Work out the finished part from the listing and answer in its coordinate system (mm). Give positions to 0.01 mm unless a question says otherwise; leave off trailing zeros. Loops run counter-clockwise (first coordinate to the right, second up) from the corner with the lowest first, then second, coordinate; pieces in that order, holes last. Notation, with made-up numbers: M 64,14.5 L 94,14.5 A20 ccw 94,42.5 Z; hole C 71.25,62 d2. An arc over 180 degrees is marked long. Write item = value, one per line. Start each with the question number.
1. Section C-C on y = -67.5 is taken. Determine the outline of the cut face in (x, z), plus the area to 3 significant figures.
2. Consider L1, parallel to X at y = -32.5, z = -9; L2, parallel to Z at x = -26, y = -16; L3, parallel to X at y = -8.5, z = -20. Determine where each line is inside the solid, lowest interval first. Write a range as [from, to].
3. Section D-D on x = 19 is taken. Determine the outline of the cut face in (y, z).
4. Flat-ended cylindrical pins translate along their axes: pin 1 Ø12 at (x, z) = (10, 13.5) entering from +Y; pin 2 Ø1.5 at (x, y) = (-49, -57.5) entering from +Z; pin 3 Ø5 at (x, y) = (41, -50.5) entering from +Z; pin 4 Ø6 at (y, z) = (-18.5, 7) entering from -X. Find the tip coordinate at first contact, or state that the pin passes through.
5. Section B-B on x = -47 is taken. Determine the outline of the cut face in (y, z), plus the area to 3 significant figures.
6. Section A-A on z = -18 is taken. Determine the outline of the cut face in (x, y), plus the area to 3 significant figures.
7. The mould has two halves that part along X. Classify faces 1 (the face through (-1, 0, -12)), 2 (the face through (-50.488, -38.633, -33.905)), 3 (the face through (-81.55, -37.57, -17.44)): released by +X, released by -X, zero draft, split by the parting line, or undercut.
```python
from build123d import *

# Parameters (mm, degrees)
F1_DEPTH = 76.2
F2_R     = 22.034775
F3_DEPTH = 254


with BuildPart() as f1:
    # F0 (on Front) → F1 (new body)
    with BuildSketch(Plane.XZ):
        with BuildLine():
            ThreePointArc((-20.306642, -38.174558), (-12.323362, -26.367866), (-9.517229, -12.394451))
            ThreePointArc((-9.517229, -12.394451), (-15.17324, 7.033301), (-30.373554, 20.389141))
            ThreePointArc((-30.373554, 20.389141), (-81.382177, -18.526161), (-20.306642, -38.174558))
        make_face()
        with BuildLine():
            ThreePointArc((-30.373554, 20.389141), (-15.17324, 7.033301), (-9.517229, -12.394451))
            ThreePointArc((-9.517229, -12.394451), (-12.323362, -26.367866), (-20.306642, -38.174558))
            Line((-20.306642, -38.174558), (60.893647, -21.640796))
            ThreePointArc((60.893647, -21.640796), (52.14333, -8.403082), (60.621694, 5.010437))
            Line((60.621694, 5.010437), (-30.373554, 20.389141))
        make_face()
        with BuildLine():
            ThreePointArc((81.371971, -8.253959), (74.628734, 4.059837), (60.621694, 5.010437))
            ThreePointArc((60.621694, 5.010437), (52.14333, -8.403082), (60.893647, -21.640796))
            ThreePointArc((60.893647, -21.640796), (74.753969, -20.486795), (81.371971, -8.253959))
        make_face()
    extrude(amount=F1_DEPTH)

    # F2 (on face) → F3 (cut)
    with BuildSketch(Plane.XZ.offset(76.2)):
        with Locations((-45.71129, -12.394451)):
            Circle(F2_R)
    extrude(amount=-F3_DEPTH, mode=Mode.SUBTRACT)


solid = f1.part
```
Verdict:
q1.outline = M -30.37,20.39 A36.19 ccw long -20.31,-38.17 L 60.89,-21.64 A14.61 ccw 81.37,-8.25 A14.61 ccw 60.62,5.01 Z; hole C -45.71,-12.39 d44.07
q1.area = 6,120 mm2
q2.L1 = [-81.75, -67.48], [-23.94, 81.35]
q2.L2 = [-42.75, -22.24], [-2.55, 19.65]
q2.L3 = [-81.1, -66.39], [-25.03, 75.45]
q3.outline = M -76.2,-30.17 L 0,-30.17 L 0,12.04 L -76.2,12.04 Z
q4.pin_1 = 0
q4.pin_2 = 23.71
q4.pin_3 = 8.75
q4.pin_4 = -77.98
q5.outline = M -76.2,-48.57 L 0,-48.57 L 0,-34.39 L -76.2,-34.39 Z; M -76.2,9.6 L 0,9.6 L 0,23.78 L -76.2,23.78 Z
q5.area = 2,160 mm2
q6.outline = M -81.47,-76.2 L -67.02,-76.2 L -67.02,0 L -81.47,0 Z; M -24.4,-76.2 L 77.65,-76.2 L 77.65,0 L -24.4,0 Z
q6.area = 8,880 mm2
q7.face_1 = zero draft
q7.face_2 = undercut
q7.face_3 = split by the parting line
